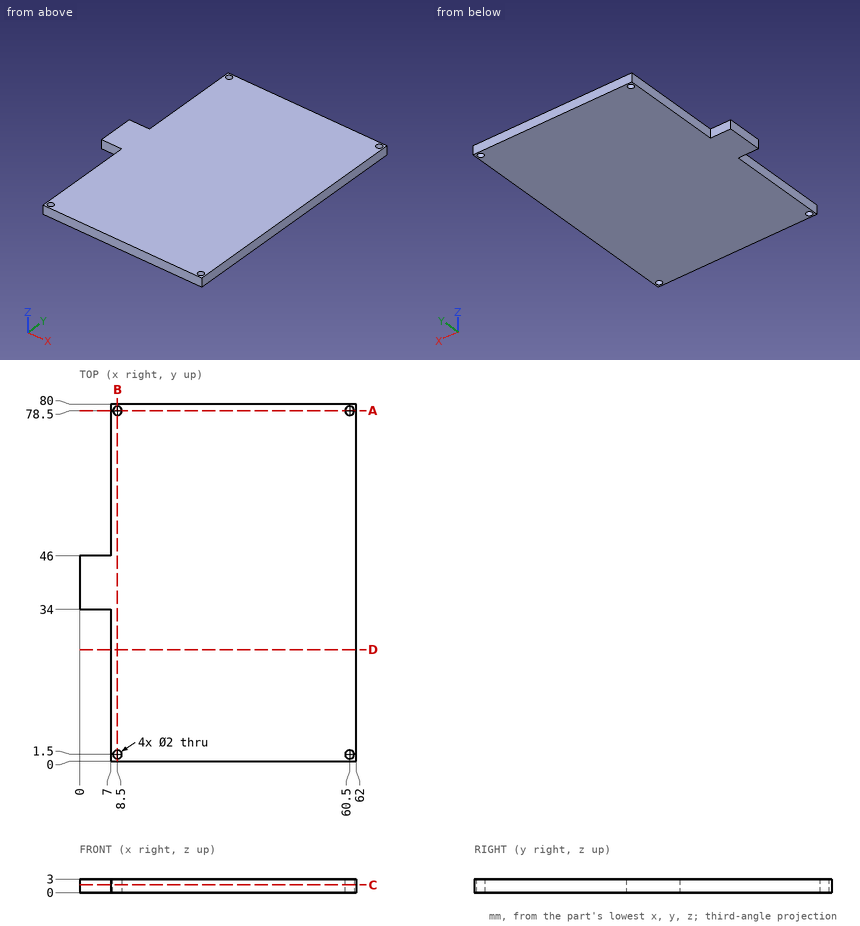
Answer from the drawing. Dimensions are ordinates in mm from the lowest x, y and z of the part. Give positions to 0.01 mm unless a question says otherwise; leave off trailing zeros. Order: outer loops, then holes, each group sorted by start corner. A loop starts at its lowest first (then second) coordinate and runs counter-clockwise, first axis right, second up. Notation, with made-up numbers: (42, -3) - (60, -3) arc R19 ccw to (60, 3) - close; hole circle Ø2 at (10, -19). An arc over 180 degrees is marked (long way). One line per item, written item: value. Start each with the question number.
1) A cutting plane is placed at A-A on y = 78.5. Give the vertices of the cut face in (x, z), then the cut area to 3 significant figures.
2) A cutting plane is placed at C-C on z = 1.7. Give the vertices of the cut face in (x, y).
3) A cutting plane is placed at B-B on x = 8.5. Give the vertices of the cut face in (y, z).
4) Given pin 1 Ø5 at (x, y) = (16.5, 49.5) entering from -Z; pin 2 Ø0.9 at (x, z) = (2, 2) entering from -Y, each flat-ended and moving along its own axis, determine where each tip first touches the part or whether it passes through.
5) Find the intervals of material crossed by L1, parallel to X at y = 78.5, z = 2.15; L2, parallel to Y at x = 60.5, z = 0.7; L3, parallel to X at y = 14, z = 1.5, in increasing order.
6) A cutting plane is placed at D-D on y = 25. Give the vertices of the cut face in (x, z), then the cut area to 3 significant figures.
Answer sheet:
1. outline: (7, 0) - (7.5, 0) - (7.5, 3) - (7, 3) - close; (9.5, 0) - (59.5, 0) - (59.5, 3) - (9.5, 3) - close; (61.5, 0) - (62, 0) - (62, 3) - (61.5, 3) - close
1. area: 153 mm2
2. outline: (0, 34) - (7, 34) - (7, 0) - (62, 0) - (62, 80) - (7, 80) - (7, 46) - (0, 46) - close; hole circle Ø2 at (8.5, 1.5); hole circle Ø2 at (8.5, 78.5); hole circle Ø2 at (60.5, 1.5); hole circle Ø2 at (60.5, 78.5)
3. outline: (0, 0) - (0.5, 0) - (0.5, 3) - (0, 3) - close; (2.5, 0) - (77.5, 0) - (77.5, 3) - (2.5, 3) - close; (79.5, 0) - (80, 0) - (80, 3) - (79.5, 3) - close
4. pin 1: stops at z = 0
4. pin 2: stops at y = 34
5. L1: x = 7 to 7.5, 9.5 to 59.5, 61.5 to 62
5. L2: y = 0 to 0.5, 2.5 to 77.5, 79.5 to 80
5. L3: x = 7 to 62
6. outline: (7, 0) - (62, 0) - (62, 3) - (7, 3) - close
6. area: 165 mm2
